CAD build for the part. Positions are in the model's coordinates, mm. Face numbers are marked on the shaded views. Round coordinates to 2 decimals unless told otherwise and drop trailing zeros. Loops run counter-clockwise (first coordinate to the right, second up) from the corner with the lowest first, then second, coordinate; pieces in that order, holes last.
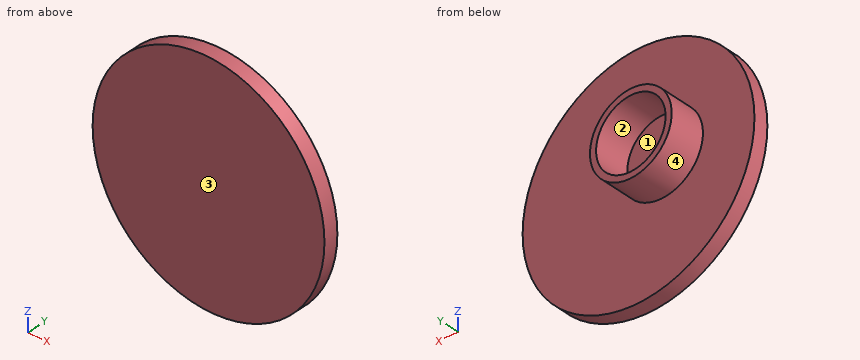
from build123d import *

# Parameters (mm, degrees)
SKETCH1_R           = 9.5
BOSS_EXTRUDE1_DEPTH = 1.2
SKETCH2_R           = 3.35
SKETCH2_R_2         = 2.85
BOSS_EXTRUDE2_DEPTH = 2.9


with BuildPart() as part:
    # Sketch1 → Boss-Extrude1 (new body)
    with BuildSketch(Plane(origin=(0, 0, 0), x_dir=(1, 0, 0), z_dir=(0, 1, 0))):
        Circle(SKETCH1_R)
    extrude(amount=BOSS_EXTRUDE1_DEPTH)

    # Sketch2 → Boss-Extrude2 (add)
    with BuildSketch(Plane(origin=(0, 1.2, 0), x_dir=(1, 0, 0), z_dir=(0, 1, 0))):
        with Locations((-1.927795475, -0.783841227)):
            Circle(SKETCH2_R)
        with Locations((-1.927795475, -0.783841227)):
            Circle(SKETCH2_R_2, mode=Mode.SUBTRACT)
    extrude(amount=BOSS_EXTRUDE2_DEPTH)


solid = part.part
Item 1: Cut at C-C (y = 1.65). List the corners of the cut face in (x, z), plus the area to 3 significant figures.
Verdict:
outline: circle Ø6.7 at (-1.93, 0.78); hole circle Ø5.7 at (-1.93, 0.78)
area: 9.74 mm2
Item 2: Mould opens along X. For the marked faces 1, 2, 3 and 4 say: released by +X, released by -X, zero draft, split by the parting line, or undercut.
Verdict:
face 1: undercut
face 2: undercut
face 3: zero draft
face 4: split by the parting line
Item 3: Cut at A-A (z = 0). List the corners of the cut face in (x, y), plus the area to 3 significant figures.
Verdict:
outline: (-9.5, 0) - (9.5, 0) - (9.5, 1.2) - (1.33, 1.2) - (1.33, 4.1) - (0.81, 4.1) - (0.81, 1.2) - (-4.67, 1.2) - (-4.67, 4.1) - (-5.18, 4.1) - (-5.18, 1.2) - (-9.5, 1.2) - close
area: 25.8 mm2
Item 4: Wall check: L1, parallel to Z at x = -0.25, y = 0.5; L2, parallel to Y at x = -1, z = -3.5; L3, parallel to X at y = 1.8, z = 1.5. Give the ranges that are in metal, low to high.
Verdict:
L1: z = -9.5 to 9.5
L2: y = 0 to 1.2
L3: x = -5.2 to -4.69, 0.83 to 1.34
Item 5: Cut at B-B (x = -4). List the corners of the cut face in (y, z), plus the area to 3 significant figures.
Verdict:
outline: (0, -8.62) - (1.2, -8.62) - (1.2, -1.85) - (4.1, -1.85) - (4.1, -1.17) - (1.2, -1.17) - (1.2, 2.74) - (4.1, 2.74) - (4.1, 3.42) - (1.2, 3.42) - (1.2, 8.62) - (0, 8.62) - close
area: 24.6 mm2
Item 6: Flat gauge pins, fed straight in: P1, Ø2, axis at x = -4.5, z = 1.5, coming from the +Y side; P2, Ø1.5, axis at y = 1, z = 3, coming from the +X side; P3, Ø2, axis at y = 0.5, z = -7.5, coming from the -X side. Where does each tip first touch, or does it go through?
Verdict:
P1: stops at y = 4.1
P2: stops at x = 9.23
P3: stops at x = -6.93
Item 7: Cut at D-D (x = 3.75). List the corners of the cut face in (y, z), plus the area to 3 significant figures.
Verdict:
outline: (0, -8.73) - (1.2, -8.73) - (1.2, 8.73) - (0, 8.73) - close
area: 20.9 mm2
